Input: part model. Units: mm. Frame: model coordinates. Give positions to 0.01 mm unless a question says otherwise; leave off trailing zeros. Loops run counter-clockwise (first coordinate to the right, second up) from the corner with the lowest first, then second, coordinate; pieces in that order, holes last.
from build123d import *

# Parameters (mm, degrees)
F1_DEPTH = 3.6
F2_R     = 3
F3_DEPTH = 3.6
F4_R     = 4
F5_DEPTH = 3.601


# Not quite as in the source:
# - a feature names something its author has since deleted; it is built from what else it names


with BuildPart() as f1:
    # F0 (on Front) → F1 (new body)
    with BuildSketch(Plane.XZ):
        with BuildLine():
            Line((50, 6), (-50, 6))
            ThreePointArc((-50, 6), (-56, 0), (-50, -6))
            Line((-50, -6), (50, -6))
            ThreePointArc((50, -6), (56, 0), (50, 6))
        make_face()
    extrude(amount=F1_DEPTH)

    # F2 (on face) → F3 (cut, through all)
    with BuildSketch(Plane.XZ.offset(3.6)):
        with Locations((-50, 0)):
            Circle(F2_R)
    extrude(amount=-F3_DEPTH, mode=Mode.SUBTRACT)

    # F4 (on face) → F5 (cut, through all)
    with BuildSketch(Plane.XZ.offset(3.6)):
        with Locations((-14, 0)):
            Circle(F4_R)
    extrude(amount=-F5_DEPTH, mode=Mode.SUBTRACT)


solid = f1.part
(1) Mould query, pull axis X, two halves, no side actions, for faces 1 (the flat face through (1, -2, 6)), 2 (the cylindrical face through (56, -2, 0)), 3 (the cylindrical face through (-18, -2, 0)). Classes: +X half, -X half, draft (parallel to the pull), parting line (faces both ways), or undercut.
Values follow:
face 1: draft
face 2: +X half
face 3: undercut
(2) Ray query, probe 1 along Z at (x, y) = (-50, -2.5); probe 2 along Z at (x, y) = (-14, -2.5); probe 3 along X at (y, z) = (-3.2, -0.75). Return the intervals inside material, ascending.
Values follow:
probe 1: z = -6 to -3, 3 to 6
probe 2: z = -6 to -4, 4 to 6
probe 3: x = -55.95 to -52.9, -47.1 to -17.93, -10.07 to 55.95
(3) Cut plane C-C (y = -2.85). Return the cut outline in (x, z), and give its area (3 significant figures).
Values follow:
outline: (-50, -6) - (50, -6) arc R6 ccw to (50, 6) - (-50, 6) arc R6 ccw to start; hole circle Ø6 at (-50, 0); hole circle Ø8 at (-14, 0)
area: 1,230 mm2
(4) Cut plane D-D (z = -5). Return the cut outline in (x, y), and give its area (3 significant figures).
Values follow:
outline: (-53.32, -3.6) - (53.32, -3.6) - (53.32, 0) - (-53.32, 0) - close
area: 384 mm2
(5) Pin query (flat end, axial travel): pin 1 Ø1 at (y, z) = (-1.5, 4) entering from -X; pin 2 Ø5.5 at (x, z) = (-50, 0) entering from -Y; pin 3 Ø2 at (y, z) = (-2, 3.5) entering from +X. Return the tip coordinate at first contact, or that it passes through.
Values follow:
pin 1: stops at x = -54.87
pin 2: passes through
pin 3: stops at x = 55.45
(6) Cut plane B-B (x = -14). Return the cut outline in (y, z).
Values follow:
outline: (-3.6, -6) - (0, -6) - (0, -4) - (-3.6, -4) - close; (-3.6, 4) - (0, 4) - (0, 6) - (-3.6, 6) - close
(7) Cut plane A-A (z = 0). Return the cut outline in (x, y), and give its area (3 significant figures).
Values follow:
outline: (-56, -3.6) - (-53, -3.6) - (-53, 0) - (-56, 0) - close; (-47, -3.6) - (-18, -3.6) - (-18, 0) - (-47, 0) - close; (-10, -3.6) - (56, -3.6) - (56, 0) - (-10, 0) - close
area: 353 mm2
